```python
from build123d import *

# Parameters (mm, degrees)
F0_W     = 25.4
F0_H     = 127
F0_R     = 5.08
F1_DEPTH = 6.35
F2_R     = 5.08
F4_DEPTH = 25.4
F6_DEPTH = 6.351


with BuildPart() as f1:
    # F0 (on Front) → F1 (new body)
    with BuildSketch(Plane.XZ):
        with Locations((0, -50.8)):
            Rectangle(F0_W, F0_H)
        Circle(F0_R, mode=Mode.SUBTRACT)
    extrude(amount=F1_DEPTH)

    # F2
    f2_edges = [f1.edges().sort_by_distance(p)[0] for p in [
        (12.7, -3.175, 12.7),
        (-12.7, -3.175, 12.7),
    ]]
    fillet(f2_edges, radius=F2_R)

    # F3 (on face) → F4 (cut)
    with BuildSketch(Plane.XZ.offset(6.35)):
        with BuildLine():
            ThreePointArc((-5.08, -41.275), (0, -46.355), (5.08, -41.275))
            Line((5.08, -41.275), (5.08, -22.225))
            ThreePointArc((5.08, -22.225), (0, -17.145), (-5.08, -22.225))
            Line((-5.08, -22.225), (-5.08, -41.275))
        make_face()
    extrude(amount=-F4_DEPTH, mode=Mode.SUBTRACT)

    # F5 (on face) → F6 (cut, through all)
    with BuildSketch(Plane.XZ.offset(6.35)):
        with BuildLine():
            Line((-5.08, -114.3), (5.08, -114.3))
            Line((5.08, -114.3), (5.08, -93.98))
            ThreePointArc((5.08, -93.98), (0, -88.9), (-5.08, -93.98))
            Line((-5.08, -93.98), (-5.08, -114.3))
        make_face()
    extrude(amount=-F6_DEPTH, mode=Mode.SUBTRACT)


solid = f1.part
```
The model under review builds one solid part; all positions refer to its coordinate system, in mm. A direction names the side the tool comes from. Round coordinates to 2 decimals unless told otherwise and drop trailing zeros. Order: outer loops, then holes, each group sorted by start corner. A loop starts at its lowest first (then second) coordinate and runs counter-clockwise, first axis right, second up.
(1) Take a section at B-B, the plane x = 0. State the section outline as (y, z) points (3 decimals).
Working result:
outline: (-6.35, -88.9) - (0, -88.9) - (0, -46.355) - (-6.35, -46.355) - close; (-6.35, -17.145) - (0, -17.145) - (0, -5.08) - (-6.35, -5.08) - close; (-6.35, 5.08) - (0, 5.08) - (0, 12.7) - (-6.35, 12.7) - close
(2) Mouldability with a two-part tool opening along X and no side actions: class faces 4 (the face through (-9, -3, -114.3)), 5 (the face through (-11.251, -3.219, 11.172)), 6 (the face through (5.08, -3, -104)) as released by +X, released by -X, zero draft, split by the parting line, or undercut.
Working result:
face 4: zero draft
face 5: released by -X
face 6: undercut
(3) Take a section at C-C, the plane z = 0. State the section outline as (x, y) points.
Working result:
outline: (-12.7, -6.35) - (-5.08, -6.35) - (-5.08, 0) - (-12.7, 0) - close; (5.08, -6.35) - (12.7, -6.35) - (12.7, 0) - (5.08, 0) - close
(4) Wall thickness on L1, parallel to Z at x = 0.5, y = -2; L2, parallel to Z at x = 0, y = -5 (3 decimals); L3, parallel to X at y = -1, z = -107: over which ranges is each line inside the solid? List them lowest first.
Working result:
L1: z = -88.92 to -46.33, -17.17 to -5.06, 5.06 to 12.7
L2: z = -88.9 to -46.355, -17.145 to -5.08, 5.08 to 12.7
L3: x = -12.7 to -5.08, 5.08 to 12.7
(5) Tool access review of faces 1 (the face through (-12.7, -3, -54)), 2 (the face through (-5.08, -3, -32)), 3 (the face through (-5.08, -3, -104)): name each direction out of +Z, -Z, +X, -X, +Y, -Y from which nothing blocks a thin tool from reaching the whole face with its end or side.
Working result:
face 1: +Z, -Z, -X, +Y, -Y
face 2: +Y, -Y
face 3: -Z, +Y, -Y
(6) For P1, Ø8, axis at x = -4.5, z = -39.5, coming from the -Y side, flat-tipped, find the tip position at first contact; note if it passes through.
Working result:
P1: stops at y = -6.35
(7) Take a section at A-A, the plane y = -3.5. State the section outline as (x, z) points (3 decimals), plus the area to 3 significant figures.
Working result:
outline: (-12.7, -114.3) - (-5.08, -114.3) - (-5.08, -93.98) arc R5.08 cw to (5.08, -93.98) - (5.08, -114.3) - (12.7, -114.3) - (12.7, 7.62) arc R5.08 ccw to (7.62, 12.7) - (-7.62, 12.7) arc R5.08 ccw to (-12.7, 7.62) - close; hole (-5.08, -41.275) arc R5.08 ccw to (5.08, -41.275) - (5.08, -22.225) arc R5.08 ccw to (-5.08, -22.225) - close; hole circle Ø10.16 at (0, 0)
area: 2,610 mm2
